from build123d import *

# Parameters (mm, degrees)
SKETCH_1_W          = 146
SKETCH_1_H          = 45
EXTRUDE_1_DEPTH     = 93
SHELL_1_T           = -1.5
SKETCH_2_W          = 28
SKETCH_2_H          = 28
CUT_EXTRUDE_1_DEPTH = 1.5
SKETCH_4_W          = 12.2
SKETCH_4_H          = 12.2
CUT_EXTRUDE_2_DEPTH = 1.5
FILLET_1_R          = 1.5


with BuildPart() as part:
    # 草图1 → 凸台-拉伸1 (new body)
    with BuildSketch(Plane(origin=(0, 0, 0), x_dir=(1, 0, 0), z_dir=(0, 1, 0))):
        Rectangle(SKETCH_1_W, SKETCH_1_H)
    extrude(amount=EXTRUDE_1_DEPTH)

    # 抽壳1
    shell_1_openings = [part.faces().sort_by_distance(p)[0] for p in [
        (0, 46.5, 22.5),
    ]]
    offset(amount=SHELL_1_T, openings=shell_1_openings, kind=Kind.INTERSECTION)

    # 草图2 → 切除-拉伸1 (cut)
    with BuildSketch(Plane.ZY.offset(73)):
        with Locations((8.5, 32.5)):
            Rectangle(SKETCH_2_W, SKETCH_2_H)
    cut_extrude_1 = extrude(amount=-CUT_EXTRUDE_1_DEPTH, mode=Mode.SUBTRACT)

    # 草图4 → 切除-拉伸2 (cut)
    with BuildSketch(Plane(origin=(0, 93, 0), x_dir=(1, 0, 0), z_dir=(0, 1, 0))):
        with Locations((0, -16.4)):
            Rectangle(SKETCH_4_W, SKETCH_4_H)
    extrude(amount=-CUT_EXTRUDE_2_DEPTH, mode=Mode.SUBTRACT)

    # 镜向1: 切除-拉伸1 across plane
    add(cut_extrude_1.mirror(Plane(origin=(0, 0, 0), x_dir=(0, 0, 1), z_dir=(1, 0, 0))), mode=Mode.SUBTRACT)

    # 圆角1
    fillet_1_edges = [part.edges().sort_by_distance(p)[0] for p in [
        (-73, 93, 0),
        (73, 93, 0),
        (-73, 0, 0),
        (0, 0, -22.5),
        (73, 0, 0),
        (-73, 46.5, -22.5),
        (73, 46.5, -22.5),
        (0, 93, -22.5),
    ]]
    fillet(fillet_1_edges, radius=FILLET_1_R)


solid = part.part
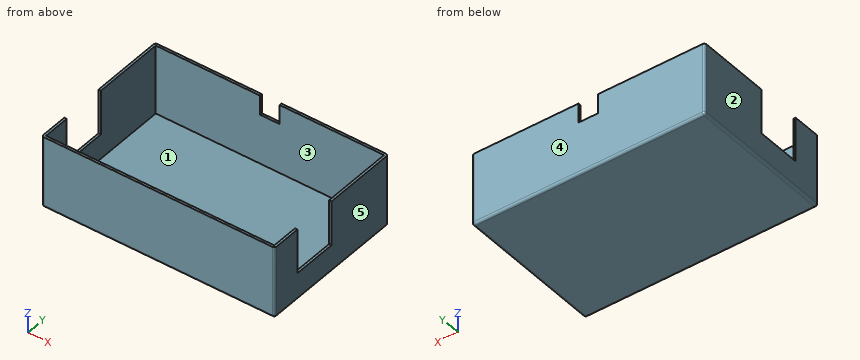
Verification items for the finished model (mm, model axes). Face numbers are marked on the shaded views. A direction names the side the tool comes from. Give positions to 0.01 mm unless a question says otherwise; leave off trailing zeros. Write each loop counter-clockwise with the first axis right and the second up, starting at its lowest first coordinate (ties: lowest second). Pieces come first, ordered by that corner, then holes.
(1) Mould release check, pull along Y, two halves, no side actions. Record for the marked faces 3, 4 and 5: +Y half, -Y half, draft (parallel to the pull), parting line (faces both ways), or undercut.
(2) Cross-section at D-D (x = -31). Enter the section's corners in (y, z).
(3) Material ranges on line 1 (X direction, y = 56, z = -16); line 2 (Y direction, x = 27, z = -11.5); line 3 (Z direction, x = -39, y = 68), recorded low to high.
(4) Access from +Z, -Z, +X, -X, +Y, -Y to the whole of each face (thin tool, end or side, straight path). Record for the marked faces 1 and 2.
(5) Cross-section at A-A (z = -1). Enter the section's corners in (x, y), plus the area to 3 significant figures.
(6) Cross-section at B-B (z = -16.5). Enter the section's corners in (x, y), plus the area to 3 significant figures.
(7) Cross-section at C-C (y = 67). Enter the section's corners in (x, z).
(8) Gauge pin test, flat ends, axial feed: pin 1 (1.6 mm diameter, centred on x = 1, y = 92, fed in from +Z); pin 2 (1.2 mm diameter, centred on x = 72, y = 36, fed in from +Z); pin 3 (5 mm diameter, centred on x = 57, y = 34.5, fed in from +Z). Record the tip position at first contact, or that the pin passes through.
Worked out:
1. face 3: undercut
1. face 4: +Y half
1. face 5: draft
2. outline: (0, -21) arc R1.5 ccw to (1.5, -22.5) - (91.5, -22.5) arc R1.5 ccw to (93, -21) - (93, 22.5) - (91.5, 22.5) - (91.5, -21) - (1.5, -21) - (1.5, 22.5) - (0, 22.5) - close
3. line 1: x = -73 to -71.5, 71.5 to 73
3. line 2: y = 0 to 1.5, 91.5 to 93
3. line 3: z = -22.5 to -21
4. face 1: +Z
4. face 2: +Z, -Z, -X, +Y, -Y
5. outline: (-73, 1.5) arc R1.5 ccw to (-71.5, 0) - (71.5, 0) arc R1.5 ccw to (73, 1.5) - (73, 18.5) - (71.5, 18.5) - (71.5, 1.5) - (-71.5, 1.5) - (-71.5, 18.5) - (-73, 18.5) - close; (-73, 46.5) - (-71.5, 46.5) - (-71.5, 91.5) - (71.5, 91.5) - (71.5, 46.5) - (73, 46.5) - (73, 91.5) arc R1.5 ccw to (71.5, 93) - (-71.5, 93) arc R1.5 ccw to (-73, 91.5) - close
5. area: 622 mm2
6. outline: (-73, 1.5) arc R1.5 ccw to (-71.5, 0) - (71.5, 0) arc R1.5 ccw to (73, 1.5) - (73, 91.5) arc R1.5 ccw to (71.5, 93) - (-71.5, 93) arc R1.5 ccw to (-73, 91.5) - close; hole (-71.5, 1.5) - (71.5, 1.5) - (71.5, 91.5) - (-71.5, 91.5) - close
6. area: 706 mm2
7. outline: (-73, -21) arc R1.5 ccw to (-71.5, -22.5) - (71.5, -22.5) arc R1.5 ccw to (73, -21) - (73, 22.5) - (71.5, 22.5) - (71.5, -21) - (-71.5, -21) - (-71.5, 22.5) - (-73, 22.5) - close
8. pin 1: stops at z = 10.3
8. pin 2: stops at z = -5.5
8. pin 3: stops at z = -21
